```python
from build123d import *

# Parameters (mm, degrees)
BOSS_EXTRUDE1_DEPTH = 11.1125
SKETCH2_R           = 3.5687
CUT_EXTRUDE1_DEPTH  = 51.8
SKETCH3_R           = 3.5687
CUT_EXTRUDE2_DEPTH  = 51.8


with BuildPart() as part:
    # Sketch1 → Boss-Extrude1 (new body, symmetric)
    with BuildSketch(Plane.XY):
        with BuildLine():
            Line((0, 0), (0, 50.8))
            ThreePointArc((0, 50.8), (3.376576302, 49.401376302), (4.7752, 46.0248))
            Line((4.7752, 46.0248), (4.7752, 7.9502))
            ThreePointArc((4.7752, 7.9502), (5.70513597, 5.70513597), (7.9502, 4.7752))
            Line((7.9502, 4.7752), (46.0248, 4.7752))
            ThreePointArc((46.0248, 4.7752), (49.401376302, 3.376576302), (50.8, 0))
            Line((50.8, 0), (0, 0))
        make_face()
    extrude(amount=BOSS_EXTRUDE1_DEPTH, both=True)

    # Sketch2 → Cut-Extrude1 (cut, through all)
    with BuildSketch(Plane(origin=(0, 0, 0), x_dir=(1, 0, 0), z_dir=(0, 1, 0))):
        with Locations((12.7, 0)):
            Circle(SKETCH2_R)
        with Locations((38.1, 0)):
            Circle(SKETCH2_R)
    extrude(amount=CUT_EXTRUDE1_DEPTH, mode=Mode.SUBTRACT)

    # Sketch3 → Cut-Extrude2 (cut, through all)
    with BuildSketch(Plane(origin=(0, 0, 0), x_dir=(0, 0, -1), z_dir=(1, 0, 0))):
        with Locations((0, 12.7)):
            Circle(SKETCH3_R)
        with Locations((0, 38.1)):
            Circle(SKETCH3_R)
    extrude(amount=CUT_EXTRUDE2_DEPTH, mode=Mode.SUBTRACT)


solid = part.part
```
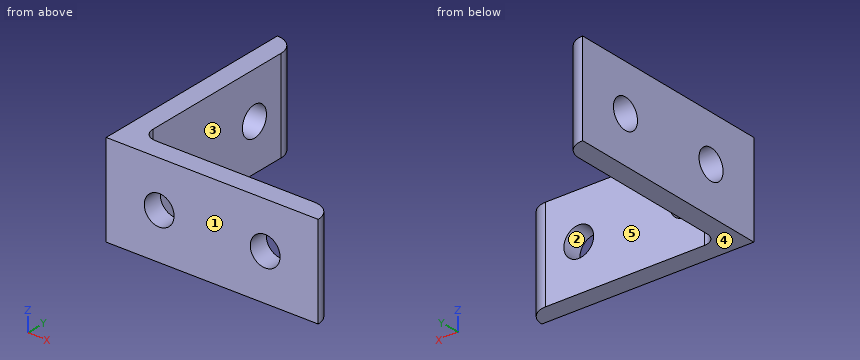
Work out the finished part from the listing and answer in its coordinate system (mm). Face numbers are marked on the shaded views. A direction names the side the tool comes from. Coordinates: 2 decimals unless noted, no trailing zeros. Order: outer loops, then holes, each group sorted by start corner. A loop starts at its lowest first (then second) coordinate and runs counter-clockwise, first axis right, second up. Notation, with made-up numbers: M 29.5,58.25 L 59.5,58.25 A23 cw 59.5,73.25 Z; hole C -29.75,28.5 d11. An arc over 180 degrees is marked long. Use CSV: the item, a comma, the result in double quotes.
1) Flat-ended cylindrical pins translate along their axes: pin 1 Ø6.5 at (y, z) = (28, -4.5) entering from +X; pin 2 Ø6.5 at (x, z) = (20.5, -2.5) entering from +Y; pin 3 Ø4.5 at (y, z) = (12.7, 0) entering from +X. Find the tip coordinate at first contact, or state that the pin passes through.
Worked out:
pin 1,"stops at x = 4.78"
pin 2,"stops at y = 4.78"
pin 3,"passes through"
2) For the marked faces 4 and 5, determine the directions among +Z, -Z, +X, -X, +Y, -Y from which every point of the face is accessible in a straight line to the end or side of a thin tool.
Worked out:
face 4,"-Z, +X, -X, +Y, -Y"
face 5,"+Z, -Z, +X, +Y"
3) Section B-B on y = 12.7 is taken. Write down the section's boundary in (x, z), plus the area to 3 significant figures.
Worked out:
outline,"M 0,-11.11 L 4.78,-11.11 L 4.78,-3.57 L 0,-3.57 Z; M 0,3.57 L 4.78,3.57 L 4.78,11.11 L 0,11.11 Z"
area,"72.0 mm^2"
4) Determine the mould class of the marked faces 1, 2 and 3 for opening direction X: released by +X, released by -X, zero draft, split by the parting line, or undercut.
Worked out:
face 1,"zero draft"
face 2,"undercut"
face 3,"released by +X"
5) Consider line 1 (Z direction, x = 38.1, y = 3.2); line 2 (X direction, y = 1.85, z = 0); line 3 (Y direction, x = 2, z = 0). Determine where each line is inside the solid, lowest interval first. Write a range as [from, to].
Worked out:
line 1,"z = [-11.11, -3.57], [3.57, 11.11]"
line 2,"x = [0, 9.13], [16.27, 34.53], [41.67, 50.43]"
line 3,"y = [0, 9.13], [16.27, 34.53], [41.67, 50.36]"
6) Section A-A on z = 0 is taken. Write down the section's boundary in (x, y) (3 decimals), plus the area to 3 significant figures.
Worked out:
outline,"M 0,0 L 9.131,0 L 9.131,4.775 L 7.95,4.775 A3.175 cw 4.775,7.95 L 4.775,9.131 L 0,9.131 Z; M 0,16.269 L 4.775,16.269 L 4.775,34.531 L 0,34.531 Z; M 0,41.669 L 4.775,41.669 L 4.775,46.025 A4.775 ccw 0,50.8 Z; M 16.269,0 L 34.531,0 L 34.531,4.775 L 16.269,4.775 Z; M 41.669,0 L 50.8,0 A4.775 ccw 46.025,4.775 L 41.669,4.775 Z"
area,"318 mm^2"
7) Section D-D on z = 6.25 is taken. Write down the section's boundary in (x, y) (3 decimals), plus the area to 3 significant figures.
Worked out:
outline,"M 0,0 L 50.8,0 A4.775 ccw 46.025,4.775 L 7.95,4.775 A3.175 cw 4.775,7.95 L 4.775,46.025 A4.775 ccw 0,50.8 Z"
area,"455 mm^2"
